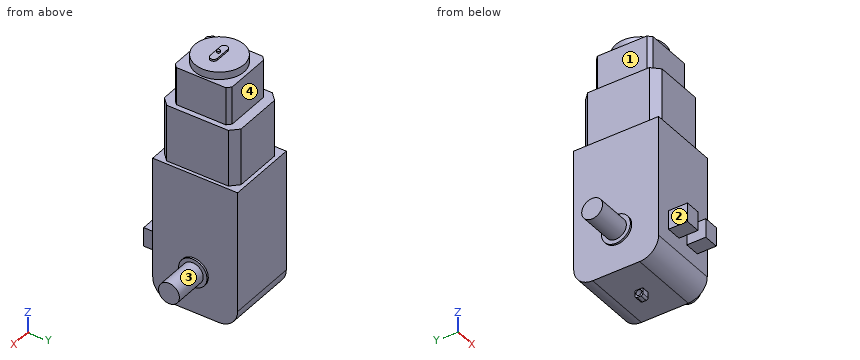
```python
from build123d import *

# Parameters (mm, degrees)
BOSS_EXTRUDE2_DEPTH      = 18.6
BOSS_EXTRUDE3_DEPTH      = 1
BOSS_EXTRUDE3_DEPTH_BACK = 1
SKETCH4_R                = 0.75
CUT_EXTRUDE1_DEPTH       = 47.139462502
BOSS_EXTRUDE5_DEPTH      = 15
BOSS_EXTRUDE6_DEPTH      = 10
SKETCH7_R                = 6.5
BOSS_EXTRUDE7_DEPTH      = 2
BOSS_EXTRUDE8_DEPTH      = 0.5
SKETCH9_R                = 0.414833025
BOSS_EXTRUDE9_DEPTH      = 0.5
SKETCH11_R               = 3.745995244
BOSS_EXTRUDE10_DEPTH     = 0.5
SKETCH13_R               = 3.818916781
BOSS_EXTRUDE11_DEPTH     = 0.5
SKETCH14_R               = 2.75
BOSS_EXTRUDE12_DEPTH     = 9.1
BOSS_EXTRUDE13_START     = 9.1
SKETCH12_R               = 2.75
BOSS_EXTRUDE13_DEPTH     = 9.1
SKETCH15_W               = 4
SKETCH15_H               = 5
BOSS_EXTRUDE14_DEPTH     = 5


with BuildPart() as part:
    # Sketch2 → Boss-Extrude2 (new body)
    with BuildSketch(Plane(origin=(0, 0, 0), x_dir=(0, 0, -1), z_dir=(1, 0, 0))):
        with BuildLine():
            Line((0, 0), (32, 0))
            ThreePointArc((32, 0), (35.535533906, -1.464466094), (37, -5))
            Line((37, -5), (37, -17.4))
            ThreePointArc((37, -17.4), (35.535533906, -20.935533906), (32, -22.4))
            Line((32, -22.4), (0, -22.4))
            Line((0, -22.4), (0, 0))
        make_face()
    extrude(amount=-BOSS_EXTRUDE2_DEPTH)

    # Sketch3 → Boss-Extrude3 (add, two sides: drawn at the far end of the back side and taken through both)
    with BuildSketch(Plane(origin=(-9.3, 0, 0), x_dir=(0, 0, -1), z_dir=(1, 0, 0)).offset(-BOSS_EXTRUDE3_DEPTH_BACK)):
        with BuildLine():
            Line((39, -11.987468366), (39, -10.987468366))
            ThreePointArc((39, -10.987468366), (38.853553391, -10.633914975), (38.5, -10.487468366))
            Line((38.5, -10.487468366), (37, -10.487468366))
            Line((37, -10.487468366), (37, -12.487468366))
            Line((37, -12.487468366), (38.5, -12.487468366))
            ThreePointArc((38.5, -12.487468366), (38.853553391, -12.341021757), (39, -11.987468366))
        make_face()
    extrude(amount=BOSS_EXTRUDE3_DEPTH + BOSS_EXTRUDE3_DEPTH_BACK)

    # Sketch4 → Cut-Extrude1 (cut, through all)
    with BuildSketch(Plane(origin=(-8.3, 0, 0), x_dir=(0, 0, -1), z_dir=(1, 0, 0))):
        with Locations((37.841364182, -11.483102308)):
            Circle(SKETCH4_R)
    extrude(amount=-CUT_EXTRUDE1_DEPTH, mode=Mode.SUBTRACT)

    # Sketch5 → Boss-Extrude5 (add)
    with BuildSketch(Plane.XY):
        Polygon((-15.706913813, -21.324455345), (-2.893086187, -21.324455345), (-0.893086187, -19.324455345), (-0.893086187, -3.075544655), (-2.893086187, -1.075544655), (-15.706913813, -1.075544655), (-17.706913813, -3.075544655), (-17.706913813, -19.324455345), align=None)
    extrude(amount=BOSS_EXTRUDE5_DEPTH)

    # Sketch6 → Boss-Extrude6 (add)
    with BuildSketch(Plane.XY.offset(15)):
        Polygon((-15.335098918, -3.69274237), (-3.264901082, -3.69274237), (-2.264901082, -4.69274237), (-2.264901082, -17.70725763), (-3.264901082, -18.70725763), (-15.335098918, -18.70725763), (-16.335098918, -17.70725763), (-16.335098918, -4.69274237), align=None)
    extrude(amount=BOSS_EXTRUDE6_DEPTH)

    # Sketch7 → Boss-Extrude7 (add)
    with BuildSketch(Plane.XY.offset(25)):
        with Locations((-9.3, -11.2)):
            Circle(SKETCH7_R)
    extrude(amount=BOSS_EXTRUDE7_DEPTH)

    # Sketch8 → Boss-Extrude8 (add)
    with BuildSketch(Plane.XY.offset(27)):
        with BuildLine():
            Line((-11.3, -10.387788461), (-7.3, -10.387788461))
            ThreePointArc((-7.3, -10.387788461), (-6.346187608, -11.341600853), (-7.3, -12.295413245))
            Line((-7.3, -12.295413245), (-11.3, -12.295413245))
            ThreePointArc((-11.3, -12.295413245), (-12.253812392, -11.341600853), (-11.3, -10.387788461))
        make_face()
    extrude(amount=BOSS_EXTRUDE8_DEPTH)

    # Sketch9 → Boss-Extrude9 (add)
    with BuildSketch(Plane.XY.offset(27.5)):
        with Locations((-9.3, -11.473161183)):
            Circle(SKETCH9_R)
    extrude(amount=BOSS_EXTRUDE9_DEPTH)

    # Sketch11 → Boss-Extrude10 (add)
    with BuildSketch(Plane(origin=(0, 0, 0), x_dir=(0, 0, -1), z_dir=(1, 0, 0))):
        with Locations((26.079029107, -11.483102308)):
            Circle(SKETCH11_R)
    extrude(amount=BOSS_EXTRUDE10_DEPTH)

    # Sketch13 → Boss-Extrude11 (add)
    with BuildSketch(Plane.ZY.offset(18.6)):
        with Locations(Location((-26.079029107, -11.483102308, 0), (0, 0, 180))):
            Circle(SKETCH13_R)
    extrude(amount=BOSS_EXTRUDE11_DEPTH)

    # Sketch14 → Boss-Extrude12 (add)
    with BuildSketch(Plane.ZY.offset(19.1)):
        with Locations((-26.079029107, -11.483102308)):
            Circle(SKETCH14_R)
    extrude(amount=BOSS_EXTRUDE12_DEPTH)

    # Sketch12 → Boss-Extrude13 (add)
    with BuildSketch(Plane(origin=(0.5, 0, 0), x_dir=(0, 0, -1), z_dir=(1, 0, 0)).offset(BOSS_EXTRUDE13_START)):
        with Locations(Location((26.079029107, -11.483102308, 0), (0, 0, 180))):
            Circle(SKETCH12_R)
    extrude(amount=-BOSS_EXTRUDE13_DEPTH)

    # Sketch15 → Boss-Extrude14 (add)
    with BuildSketch(Plane.XZ.offset(22.4)):
        with Locations((-5.8, -25.582825972)):
            Rectangle(SKETCH15_W, SKETCH15_H)
        with Locations((-12.8, -25.582825972)):
            Rectangle(SKETCH15_W, SKETCH15_H)
    extrude(amount=BOSS_EXTRUDE14_DEPTH)


solid = part.part
```
Can you work these out from the model? Positions are in its coordinate system, mm. Face numbers are marked on the shaded views. A direction names the side the tool comes from. Coordinates: 2 decimals unless noted, no trailing zeros. Loops run counter-clockwise (first coordinate to the right, second up) from the corner with the lowest first, then second, coordinate; pieces in that order, holes last. Notation, with made-up numbers: (8.25, 3.25) - (57.25, 3.25) arc R21 ccw to (57.25, 42.25) - close; hole circle Ø8 at (-13, -27). An arc over 180 degrees is marked (long way). Answer as CSV lines item,"result". Start each with the question number.
1) Suppose I cut it at D-D (y = -20.5). Please give me the cut outline in (x, z), plus the area to 3 significant figures.
2) For pin 1 (5.5 mm diameter, centred on y = -26, z = -24.5, fed in from -X); pin 2 (0.9 mm diameter, centred on y = -11.48, z = -37.84, fed in from -X); pin 3 (2 mm diameter, centred on y = -6, z = -6, fed in from +X); pin 4 (2 mm diameter, centred on x = -3.5, y = -12.5, fed in from -Z), each with a flat end and sliding along its axis, tell me the tip position at first contact or that it passes through.
3) Suppose I cut it at A-A (y = -25.25). Please give me the cut outline in (x, z), plus the area to 3 significant figures.
4) I need wall thicknesses on line 1 (Y direction, x = -17.5, z = -6); line 2 (X direction, y = -23, z = -26); line 3 (Y direction, x = -10.5, z = 12.5). Which ranges of each line are inside material? Lowest first, please. Write a range as from..to.
5) Suppose I cut it at B-B (z = 3.5). Please give me the cut outline in (x, y).
6) Suppose I cut it at C-C (x = -13). Please give me the cut outline in (y, z), plus the area to 3 significant figures.
7) Which directions (+Z, -Z, +X, -X, +Y, -Y) give clear straight access to the entire face, cutting with the end or side of a thin tool? Please do the marked faces 1, 2, 3 and 4.
Check result:
1,outline,"(-18.6, -35.92) - (0, -35.92) - (0, 0) - (-2.07, 0) - (-2.07, 15) - (-16.53, 15) - (-16.53, 0) - (-18.6, 0) - close"
1,area,"885 mm²"
2,pin 1,"stops at x = -14.8"
2,pin 2,"passes through"
2,pin 3,"stops at x = 0"
2,pin 4,"stops at z = -37"
3,outline,"(-14.8, -28.08) - (-10.8, -28.08) - (-10.8, -23.08) - (-14.8, -23.08) - close; (-7.8, -28.08) - (-3.8, -28.08) - (-3.8, -23.08) - (-7.8, -23.08) - close"
3,area,"40.0 mm²"
4,line 1,"y = -22.4..0"
4,line 2,"x = -14.8..-10.8, -7.8..-3.8"
4,line 3,"y = -21.32..-1.08"
5,outline,"(-17.71, -19.32) - (-15.71, -21.32) - (-2.89, -21.32) - (-0.89, -19.32) - (-0.89, -3.08) - (-2.89, -1.08) - (-15.71, -1.08) - (-17.71, -3.08) - close"
6,outline,"(-27.4, -28.08) - (-22.4, -28.08) - (-22.4, -32) arc R5 ccw to (-17.4, -37) - (-5, -37) arc R5 ccw to (0, -32) - (0, 0) - (-1.08, 0) - (-1.08, 15) - (-3.69, 15) - (-3.69, 25) - (-5.86, 25) - (-5.86, 27) - (-16.54, 27) - (-16.54, 25) - (-18.71, 25) - (-18.71, 15) - (-21.32, 15) - (-21.32, 0) - (-22.4, 0) - (-22.4, -23.08) - (-27.4, -23.08) - close"
6,area,"1,320 mm²"
7,face 1,"+Z, -X, +Y, -Y"
7,face 2,"+Z, -Z, -X, -Y"
7,face 3,"+X"
7,face 4,"+Z, +X, -X, +Y"
